```python
from build123d import *

# Parameters (mm, degrees)
BOSS_EXTRUDE1_DEPTH                 = 25.4
SHELL1_T                            = -3.175
SKETCH4_R                           = 12.7
BOSS_EXTRUDE3_DEPTH                 = 19.05
BOSS_EXTRUDE4_DEPTH                 = 19.05
SKETCH6_R                           = 12.7
CUT_EXTRUDE2_DEPTH                  = 12.7
CUT_EXTRUDE3_START                  = 12.7
SKETCH6_2_R                         = 12.7
CUT_EXTRUDE3_DEPTH                  = 12.7
CUT_EXTRUDE4_REACH                  = 98.093
SKETCH7_R                           = 3.175
BOSS_EXTRUDE5_REACH                 = 98.093
CUT_EXTRUDE5_DEPTH                  = 12.7
BOSS_EXTRUDE6_DEPTH                 = 25.4
FILLET2_R                           = 12.7
CUT_EXTRUDE6_REACH                  = 109.812
CUT_EXTRUDE6_END_RADIUS             = 3.175
SKETCH12_R                          = 1.7526
CUT_EXTRUDE6_DIRECTION_2_REACH      = 109.812
CUT_EXTRUDE6_DIRECTION_2_END_RADIUS = 12.7


with BuildPart() as part:
    # Sketch2 → Boss-Extrude1 (new, symmetric)
    with BuildSketch(Plane(origin=(0, 0, 0), x_dir=(0, 0, -1), z_dir=(1, 0, 0))):
        with BuildLine():
            Line((0, 0), (0, 76.2))
            ThreePointArc((0, 76.2), (-38.1, 38.1), (0, 0))
        make_face()
    extrude(amount=BOSS_EXTRUDE1_DEPTH, both=True)

    # Shell1
    shell1_openings = [part.faces().sort_by_distance(p)[0] for p in [
        (0, 38.1, 0),
    ]]
    offset(amount=SHELL1_T, openings=shell1_openings)



with BuildPart() as body_2:
    # Sketch4 → Boss-Extrude3 (new, symmetric)
    with BuildSketch(Plane(origin=(0, 0, 0), x_dir=(0, 0, -1), z_dir=(1, 0, 0))):
        with Locations(Location((9.525, -9.525, 0), (0, 0, 180))):
            Circle(SKETCH4_R)
    extrude(amount=BOSS_EXTRUDE3_DEPTH, both=True)


with BuildPart() as part_1:
    add(part.part)

    add(body_2.part)  # Boss-Extrude4 merges body 2
    # Sketch5 → Boss-Extrude4 (add, symmetric)
    with BuildSketch(Plane(origin=(0, 0, 0), x_dir=(0, 0, -1), z_dir=(1, 0, 0))):
        with BuildLine():
            Line((0, 3.175), (0, 0))
            Line((0, 0), (1.124739587, 0))
            ThreePointArc((1.124739587, 0), (5.034871939, 2.354762203), (9.525, 3.175))
            Line((9.525, 3.175), (0, 3.175))
        make_face()
    extrude(amount=BOSS_EXTRUDE4_DEPTH, both=True)

    # Sketch6 → Cut-Extrude2 (cut)
    with BuildSketch(Plane(origin=(0, 0, 0), x_dir=(0, 0, -1), z_dir=(1, 0, 0))):
        with Locations((9.525, -9.525)):
            Circle(SKETCH6_R)
    extrude(amount=-CUT_EXTRUDE2_DEPTH, mode=Mode.SUBTRACT)

    # Sketch6<2> → Cut-Extrude3 (cut)
    with BuildSketch(Plane(origin=(0, 0, 0), x_dir=(0, 0, -1), z_dir=(1, 0, 0)).offset(CUT_EXTRUDE3_START)):
        with Locations((9.525, -9.525)):
            Circle(SKETCH6_2_R)
    extrude(amount=-CUT_EXTRUDE3_DEPTH, mode=Mode.SUBTRACT)

    # Cut-Extrude4: up to this face of the body (flat: up to its plane)
    cut_extrude4_end = Plane(part_1.part.faces().sort_by_distance((19.05, -9.258016607, -9.360446087))[0])
    # Sketch7 → Cut-Extrude4 (cut, up to the picked face)
    with BuildSketch(Plane.ZY.offset(19.05), mode=Mode.PRIVATE) as cut_extrude4_sk1:
        with Locations(Location((-9.525, -9.525, 0), (0, 0, 180))):
            Circle(SKETCH7_R)
    cut_extrude4_tool1 = split(extrude(cut_extrude4_sk1.sketch, amount=-CUT_EXTRUDE4_REACH, mode=Mode.PRIVATE), bisect_by=cut_extrude4_end, keep=Keep.BOTH, mode=Mode.PRIVATE)
    add(cut_extrude4_tool1.solids().sort_by(Axis((-19.05, -9.525, -9.525), (1, 0, 0)))[0], mode=Mode.SUBTRACT)

    # Boss-Extrude5: up to this face of the body (flat: up to its plane)
    boss_extrude5_end = Plane(part_1.part.faces().sort_by_distance((-19.05, 2.815789755, -4.7625))[0])
    # Sketch8 → Boss-Extrude5 (add, up to the picked face)
    with BuildSketch(Plane(origin=(19.05, 0, 0), x_dir=(0, 0, -1), z_dir=(1, 0, 0)), mode=Mode.PRIVATE) as boss_extrude5_sk1:
        with BuildLine():
            Line((-27.936104056, 12.192779189), (0.212965315, -18.16074027))
            Line((0.212965315, -18.16074027), (5.034871939, -21.404762203))
            Line((5.034871939, -21.404762203), (1.124739587, 0))
            Line((1.124739587, 0), (0, 3.175))
            ThreePointArc((0, 3.175), (-13.704863106, 5.9762961), (-25.211222013, 13.9308066))
            Line((-25.211222013, 13.9308066), (-27.936104056, 12.192779189))
        make_face()
    boss_extrude5_tool1 = split(extrude(boss_extrude5_sk1.sketch, amount=-BOSS_EXTRUDE5_REACH, mode=Mode.PRIVATE), bisect_by=boss_extrude5_end, keep=Keep.BOTH, mode=Mode.PRIVATE)
    add(boss_extrude5_tool1.solids().sort_by(Axis((19.05, -2.840531, 7.724646), (-1, 0, 0)))[0])

    # Sketch9 → Cut-Extrude5 (cut, symmetric)
    with BuildSketch(Plane(origin=(0, 0, 0), x_dir=(0, 0, -1), z_dir=(1, 0, 0))):
        with BuildLine():
            Line((0, 3.175), (0, 0))
            ThreePointArc((0, 0), (-15.240486985, 3.180985746), (-27.936104056, 12.192779189))
            Line((-27.936104056, 12.192779189), (0.212965315, -18.16074027))
            ThreePointArc((0.212965315, -18.16074027), (21.164671418, -14.605162328), (9.525, 3.175))
            Line((9.525, 3.175), (0, 3.175))
        make_face()
    extrude(amount=CUT_EXTRUDE5_DEPTH, both=True, mode=Mode.SUBTRACT)

    # Sketch11 → Boss-Extrude6 (add, symmetric)
    with BuildSketch(Plane(origin=(0, 0, 0), x_dir=(0, 0, -1), z_dir=(1, 0, 0))):
        Polygon((2.609832197, 76.2), (0, 76.2), (0, 73.025), align=None)
    extrude(amount=BOSS_EXTRUDE6_DEPTH, both=True)

    # Fillet2
    # the kernel refuses this fillet: 12.7 mm, written as the material it adds along each edge
    with BuildSketch(Plane(origin=(-22.225, 38.1, 0), x_dir=(0, 1, 0), z_dir=(0, 0, -1))) as fillet2_piece_1:
        with BuildLine():
            CenterArc((34.925 - FILLET2_R, FILLET2_R), FILLET2_R, 270, 90)
            Line((34.925 - FILLET2_R, 0), (34.925, 0))
            Line((34.925, 0), (34.925, FILLET2_R))
        make_face()
    revolve(axis=Axis((-22.225, 38.1, 0), (1, 0, 0)), revolution_arc=180)
    with BuildSketch(Plane(origin=(22.225, 38.1, 0), x_dir=(0, 1, 0), z_dir=(0, 0, -1))) as fillet2_piece_2:
        with BuildLine():
            CenterArc((34.925 - FILLET2_R, -FILLET2_R), FILLET2_R, 0, 90)
            Line((34.925 - FILLET2_R, 0), (34.925, 0))
            Line((34.925, 0), (34.925, -FILLET2_R))
        make_face()
    revolve(axis=Axis((22.225, 38.1, 0), (1, 0, 0)), revolution_arc=180)

    # Cut-Extrude6: up to this cylinder (the profile starts outside it)
    cut_extrude6_end = Plane(origin=(0, -9.525, -9.525), z_dir=(-1, 0, 0)) * Cylinder(CUT_EXTRUDE6_END_RADIUS, 258.724, mode=Mode.PRIVATE)
    # Sketch12 → Cut-Extrude6 (cut, up to the surface)
    with BuildSketch(Plane(origin=(0, -21.404762203, 0), x_dir=(1, 0, 0), z_dir=(0, 1, 0)), mode=Mode.PRIVATE) as cut_extrude6_sk1:
        with Locations(Location((15.875, 9.525, 0), (0, 0, 90))):
            Circle(SKETCH12_R)
    cut_extrude6_tool1 = extrude(cut_extrude6_sk1.sketch, amount=CUT_EXTRUDE6_REACH, mode=Mode.PRIVATE) - cut_extrude6_end
    add(cut_extrude6_tool1.solids().sort_by_distance((15.875, -21.404762, -9.525))[0], mode=Mode.SUBTRACT)
    # Sketch12 → Cut-Extrude6 (cut, up to the surface)
    with BuildSketch(Plane(origin=(0, -21.404762203, 0), x_dir=(1, 0, 0), z_dir=(0, 1, 0)), mode=Mode.PRIVATE) as cut_extrude6_sk2:
        with Locations(Location((-15.875, 9.525, 0), (0, 0, 90))):
            Circle(SKETCH12_R)
    cut_extrude6_tool2 = extrude(cut_extrude6_sk2.sketch, amount=CUT_EXTRUDE6_REACH, mode=Mode.PRIVATE) - cut_extrude6_end
    add(cut_extrude6_tool2.solids().sort_by_distance((-15.875, -21.404762, -9.525))[0], mode=Mode.SUBTRACT)

    # Cut-Extrude6 direction 2: up to this cylinder (the profile starts inside it)
    cut_extrude6_direction_2_end = Plane(origin=(0, -9.525, -9.525), z_dir=(-1, 0, 0)) * Cylinder(CUT_EXTRUDE6_DIRECTION_2_END_RADIUS, 277.774, mode=Mode.PRIVATE)
    # Sketch12 → Cut-Extrude6 direction 2 (cut, up to the surface)
    with BuildSketch(Plane(origin=(0, -21.404762203, 0), x_dir=(1, 0, 0), z_dir=(0, 1, 0)), mode=Mode.PRIVATE) as cut_extrude6_direction_2_sk1:
        with Locations(Location((15.875, 9.525, 0), (0, 0, 90))):
            Circle(SKETCH12_R)
    cut_extrude6_direction_2_tool1 = extrude(cut_extrude6_direction_2_sk1.sketch, amount=-CUT_EXTRUDE6_DIRECTION_2_REACH, mode=Mode.PRIVATE) & cut_extrude6_direction_2_end
    add(cut_extrude6_direction_2_tool1.solids().sort_by_distance((15.875, -21.404762, -9.525))[0], mode=Mode.SUBTRACT)
    # Sketch12 → Cut-Extrude6 direction 2 (cut, up to the surface)
    with BuildSketch(Plane(origin=(0, -21.404762203, 0), x_dir=(1, 0, 0), z_dir=(0, 1, 0)), mode=Mode.PRIVATE) as cut_extrude6_direction_2_sk2:
        with Locations(Location((-15.875, 9.525, 0), (0, 0, 90))):
            Circle(SKETCH12_R)
    cut_extrude6_direction_2_tool2 = extrude(cut_extrude6_direction_2_sk2.sketch, amount=-CUT_EXTRUDE6_DIRECTION_2_REACH, mode=Mode.PRIVATE) & cut_extrude6_direction_2_end
    add(cut_extrude6_direction_2_tool2.solids().sort_by_distance((-15.875, -21.404762, -9.525))[0], mode=Mode.SUBTRACT)


solid = part_1.part
```
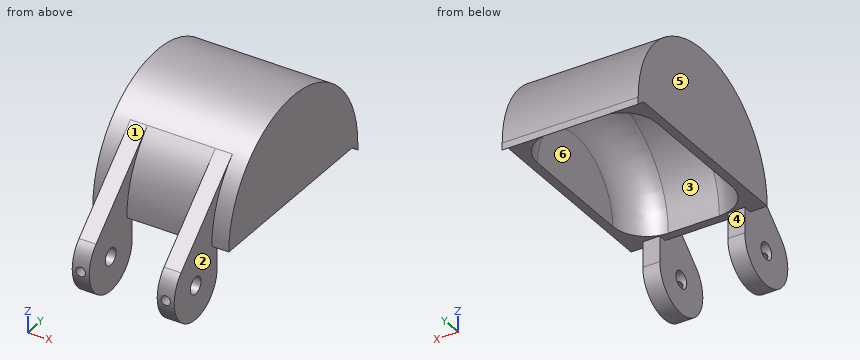
The model under review builds one solid part; all positions refer to its coordinate system, in mm. Face numbers are marked on the shaded views. A direction names the side the tool comes from. Give positions to 0.01 mm unless a question says otherwise; leave off trailing zeros. Loops run counter-clockwise (first coordinate to the right, second up) from the corner with the lowest first, then second, coordinate; pieces in that order, holes last. Notation, with made-up numbers: (25.5, 23) - (44.5, 23) arc R29 cw to (44.5, 47) - close; hole circle Ø8 at (-6, 20). An arc over 180 degrees is marked (long way). Answer as a JSON object with one key per item and string values.
Q1. Insertion check: pin 1 (2 mm diameter, centred on x = -12.5, z = -5.5, fed in from +Y) (3 decimals); pin 2 (5 mm diameter, centred on x = -13, y = -2, fed in from -Z); pin 3 (10 mm diameter, centred on x = 17, z = 4, fed in from -Y); pin 4 (5 mm diameter, centred on y = -9.525, z = -9.525, fed in from +X). Each pin has a flat end and moves straight along its axis. Give the tip position at first contact, or say it passes through.
Worked out:
{"pin 1": "stops at y = 3.175", "pin 2": "stops at z = -21.19", "pin 3": "stops at y = -18.94", "pin 4": "passes through"}
Q2. Add section B-B on x = -6.5. State the section outline as (y, z) points (3 decimals), plus the area to 3 significant figures.
Worked out:
{"outline": "(0, 0) - (3.175, 0) arc R34.925 cw to (73.025, 0) - (76.2, -2.61) - (76.2, 0) arc R38.1 ccw to start", "area": "368 mm^2"}
Q3. Mouldability with a two-part tool opening along Y and no side actions: class the marked faces 1, 2 and 3 as +Y half, -Y half, draft (parallel to the pull), parting line (faces both ways), or undercut.
Worked out:
{"face 1": "-Y half", "face 2": "draft", "face 3": "undercut"}
Q4. To check wall thickness, follow line 1 along X through (y, z) = (-1.5, -14); line 2 along X through (y, z) = (44, 7.5) (3 decimals); line 3 along X through (y, z) = (-13, -9). State the ranges of each line that lie inside material, in increasing order.
Worked out:
{"line 1": "x = -19.05 to -12.7, 12.7 to 19.05", "line 2": "x = -25.4 to -22.225, 22.225 to 25.4", "line 3": "x = -19.05 to -17.55, -14.2 to -12.7, 12.7 to 14.2, 17.55 to 19.05"}
Q5. Add section A-A on y = 38.1. State the section outline as (x, z) points (3 decimals), plus the area to 3 significant figures.
Worked out:
{"outline": "(-25.4, 0) - (-22.225, 0) - (-22.225, 22.225) arc R12.7 cw to (-9.525, 34.925) - (9.525, 34.925) arc R12.7 cw to (22.225, 22.225) - (22.225, 0) - (25.4, 0) - (25.4, 38.1) - (-25.4, 38.1) - close", "area": "452 mm^2"}
Q6. For the marked faces 4, 5 and 6, list the 3-axis set-ups (+Z, -Z, +X, -X, +Y, -Y) from which the entire face can be reached by the end or side of a thin tool; tool diameter is ignored.
Worked out:
{"face 4": "-Z, +X, -X", "face 5": "+Z, -Z, -X, +Y, -Y", "face 6": "-Z"}
